Input: dimensioned drawing with shaded views. Units: mm. Origin: part minimum x, y, z. A direction names the side the tool comes from. Give positions to 0.01 mm unless a question says otherwise; leave off trailing zeros. Write each loop counter-clockwise with the first axis right and the second up, starting at its lowest first coordinate (ties: lowest second). Pieces come first, ordered by that corner, then holes.
Q1. Reachability of the marked faces 1 and 2 from +Z, -Z, +X, -X, +Y, -Y: full face, straight path, thin tool, end or side. Return the list, or none.
Q2. Section B-B (z = 256.5). Return the cut outline in (x, y) (3 decimals).
Q3. Line query: line 1 (Z direction, x = 42.5, y = 19.5); line 2 (Y direction, x = 36, z = 71.5); line 3 (Z direction, x = 63, y = 52). Output: solid intervals per line, ascending.
Q4. Pin query (flat end, axial travel): pin 1 Ø1.5 at (x, y) = (16.5, 62.5) entering from -Z; pin 2 Ø8 at (x, y) = (11.5, 10) entering from +Z; pin 3 Ø8 at (x, z) = (24, 50) entering from -Y. Return the tip coordinate at first contact, or that it passes through.
Q5. Section A-A (z = 289). Return the cut outline in (x, y) (3 decimals).
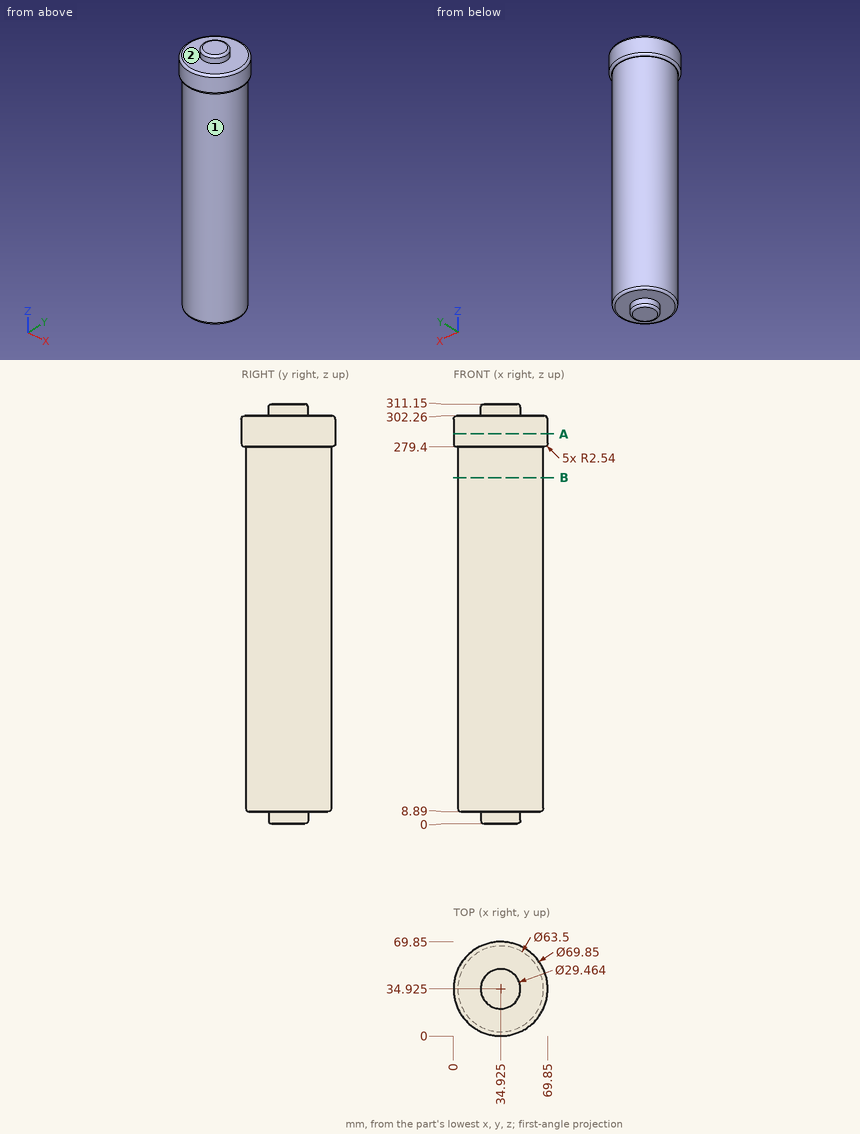
Computed:
1. face 1: -Z
1. face 2: +Z
2. outline: circle Ø63.5 at (34.925, 34.925)
3. line 1: z = 8.89 to 302.26
3. line 2: y = 3.19 to 66.66
3. line 3: z = 279.44 to 302.22
4. pin 1: stops at z = 279.4
4. pin 2: stops at z = 302.26
4. pin 3: stops at y = 3.94
5. outline: circle Ø69.85 at (34.925, 34.925)
